Design review of the part shown in the three views and the two pictorial views. Dimensions are in mm from the part's minimum x, y and z. A direction names the side the tool comes from. Round coordinates to 2 decimals unless told otherwise and drop trailing zeros. Order: outer loops, then holes, each group sorted by start corner. A loop starts at its lowest first (then second) coordinate and runs counter-clockwise, first axis right, second up. Notation, with made-up numbers: (-32.5, 69) - (14.5, 69) arc R32 ccw to (14.5, 104) - close; hole circle Ø5 at (-14, 50). An arc over 180 degrees is marked (long way). Use CSV: the item, a comma, the result in double quotes.
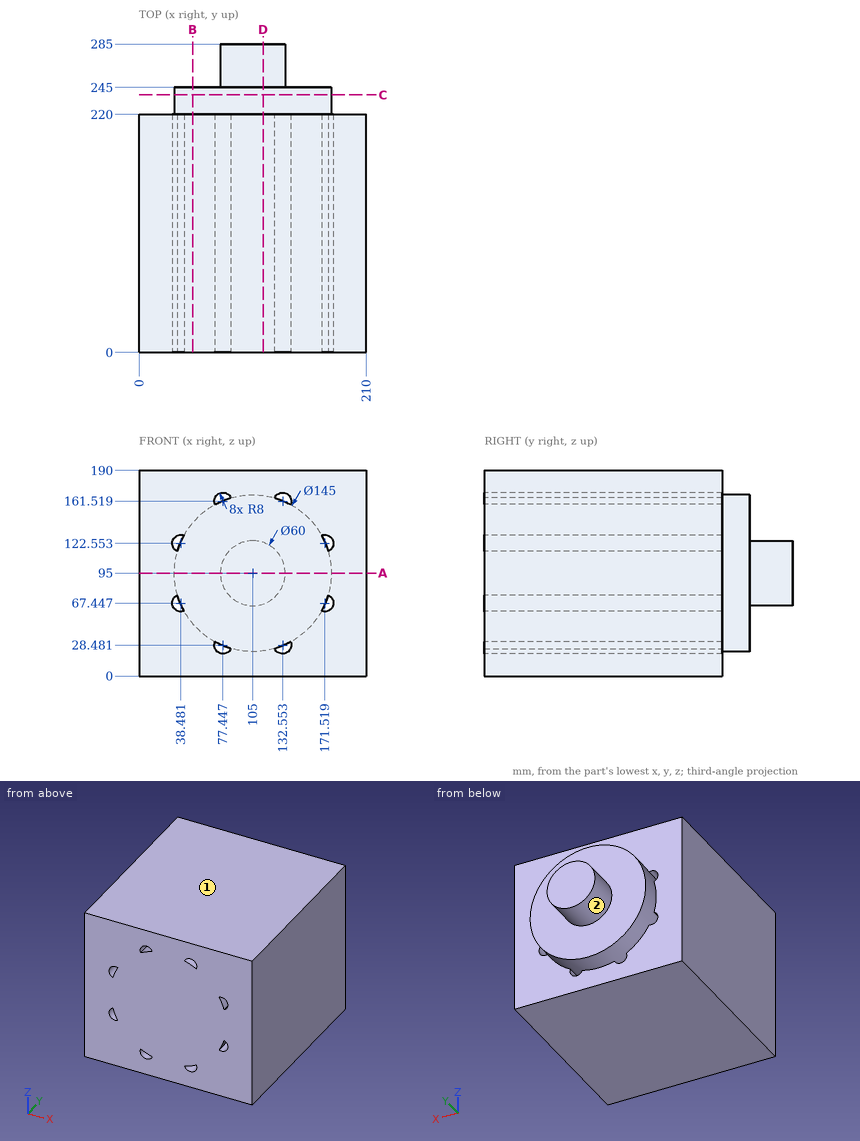
1) We need section C-C (y = 238). Give the boundary of the cut face in (x, z), then the cut area to 3 significant figures.
Data:
outline,"circle Ø145 at (105, 95)"
area,"16,500 mm2"
2) For the marked faces 1 and 2, list the 3-axis set-ups (+Z, -Z, +X, -X, +Y, -Y) from which the entire face can be reached by the end or side of a thin tool; tool diameter is ignored.
Data:
face 1,"+Z, +X, -X, +Y, -Y"
face 2,"+Y"
3) We need section B-B (x = 49.5). Give the boundary of the cut face in (y, z), then the cut area to 3 significant figures.
Data:
outline,"(0, 0) - (220, 0) - (220, 48.35) - (245, 48.35) - (245, 141.65) - (220, 141.65) - (220, 190) - (0, 190) - close"
area,"44,100 mm2"
4) To check wall thickness, follow L1, parallel to X at y = 79.5, z = 160 (1 decimal); L2, parallel to X at y = 12.5, z = 159.5 (1 decimal); L3, parallel to Y at x = 23.5, z = 159.5. State the ranges of each line that lie inside material, in increasing order. Write a range as from..to.
Data:
L1,"x = 0..69.6, 72.9..137.1, 140.4..210"
L2,"x = 0..69.7, 71.9..138.1, 140.3..210"
L3,"y = 0..220"
5) Insertion check: pin 1 Ø10 at (y, z) = (211, 30.5) entering from -X; pin 2 Ø12 at (x, y) = (81, 232) entering from -Z; pin 3 Ø8 at (x, z) = (135.5, 39.5) entering from +Y. Each pin has a flat end and moves straight along its axis. Give the tip position at first contact, or say it passes through.
Data:
pin 1,"stops at x = 0"
pin 2,"stops at z = 24.77"
pin 3,"stops at y = 245"
6) We need section D-D (x = 114.5). Give the boundary of the cut face in (y, z) (1 decimal), then the cut area to 3 significant figures.
Data:
outline,"(0, 0) - (220, 0) - (220, 23.1) - (245, 23.1) - (245, 66.5) - (285, 66.5) - (285, 123.5) - (245, 123.5) - (245, 166.9) - (220, 166.9) - (220, 190) - (0, 190) - close"
area,"47,700 mm2"
7) We need section A-A (z = 95). Give the boundary of the cut face in (x, y).
Data:
outline,"(0, 0) - (210, 0) - (210, 220) - (177.5, 220) - (177.5, 245) - (135, 245) - (135, 285) - (75, 285) - (75, 245) - (32.5, 245) - (32.5, 220) - (0, 220) - close"
